```python
from build123d import *

# Parameters (mm, degrees)
F0_W     = 5.08
F0_H     = 5.08
F1_DEPTH = 2.54
F4_W     = 1.27
F4_H     = 3.048
F5_DEPTH = 5.08
F3_W     = 2.921
F3_H     = 1.27


with BuildPart() as f1:
    # F0 (on Right) → F1 (new body, symmetric)
    with BuildSketch(Plane.YZ):
        Rectangle(F0_W, F0_H)
    extrude(amount=F1_DEPTH, both=True)

    # F4 (on face) → F5 (cut, through all)
    with BuildSketch(Plane.YZ.offset(2.54)):
        Rectangle(F4_W, F4_H)
    extrude(amount=-F5_DEPTH, mode=Mode.SUBTRACT)

    # F6: sweep along a path in F2
    with BuildLine(Plane.XZ) as f6_path:
        Line((0, -2.54), (0, -6.096))
        Line((0, -6.096), (-10.541, -6.096))
        Line((-10.541, -6.096), (-10.541, 0))
        Line((-10.541, 0), (7.8415209427, 0))
    # F3 (on face) → F6 (sweep)
    with BuildSketch(Plane(origin=(0, 0, -2.54), x_dir=(1, 0, 0), z_dir=(0, 0, -1))):
        Rectangle(F3_W, F3_H)
    sweep(path=f6_path.line, transition=Transition.RIGHT)


solid = f1.part
```
Check sheet for the modelled part. Datum: model origin and axes. Units: mm. A direction names the side the tool comes from. Round coordinates to 2 decimals unless told otherwise and drop trailing zeros. Order: outer loops, then holes, each group sorted by start corner. A loop starts at its lowest first (then second) coordinate and runs counter-clockwise, first axis right, second up. Notation, with made-up numbers: (-14, 6.5) -> (1, 6.5) arc R3 cw to (1, 10.5) -> close; hole circle Ø11 at (70.25, -9). An arc over 180 degrees is marked (long way). One line per item, written item: value. Start each with the question number.
Q1. Cross-section at A-A (x = -4). Record the boundary of the cut face in (y, z) (1 decimal).
Q2. Thickness scan on line 1 (X direction, y = -0.25, z = -2); line 2 (Y direction, x = -9, z = -0.25) (3 decimals); line 3 (Z direction, x = -4.5, y = 0.35). Record the ranges inside material, lowest first.
Q3. Mould release check, pull along Z, two halves, no side actions. Record for faces 6 (the face through (-5, 0, -7.556)), 7 (the face through (-5, 0, -4.636)), 8 (the face through (-1.46, 0, -4)), 9 (the face through (-7, -0.635, -5)): pulls with the +Z half, pulls with the -Z half, needs draft (parallel to the pull), parting line crosses it, or undercut.
Q4. Cross-section at B-B (y = -0.2). Record the boundary of the cut face in (x, z).
Q5. Cross-section at D-D (x = -0.25). Give the number of separate pieces and of enclosed holes in the cut face, and give its area (3 significant figures).
Q6. Cross-section at C-C (z = -1). Record the boundary of the cut face in (x, y) (1 decimal).
Q7. Gauge pin test, flat ends, axial feed: pin 1 Ø4.5 at (x, z) = (-8, -2.5) entering from -Y (3 decimals); pin 2 Ø1 at (y, z) = (0.5, -4.5) entering from +X; pin 3 Ø1 at (x, y) = (4, -1) entering from +Z. Record the tip position at first contact, or that the pin passes through.
Q8. Set-up check for faces 1 (the face through (1.46, 0, -5)), 2 (the face through (-7, 0.635, -5)), 3 (the face through (-9.08, 0, -3)), 4 (the face through (5, -0.635, 0)), 5 (the face through (5, 0.635, 0)): record each of +Z, -Z, +X, -X, +Y, -Y from which the full face is reachable in a straight line by a thin tool's end or side.
Completed:
1. outline: (-0.6, -7.6) -> (0.6, -7.6) -> (0.6, -4.6) -> (-0.6, -4.6) -> close; (-0.6, -1.5) -> (0.6, -1.5) -> (0.6, 1.5) -> (-0.6, 1.5) -> close
2. line 1: x = -12 to -9.08, -2.54 to 2.54
2. line 2: y = -0.635 to 0.635
2. line 3: z = -7.56 to -4.64, -1.46 to 1.46
3. face 6: pulls with the -Z half
3. face 7: undercut
3. face 8: undercut
3. face 9: needs draft
4. outline: (-12, -7.56) -> (1.46, -7.56) -> (1.46, -2.54) -> (2.54, -2.54) -> (2.54, -1.52) -> (-2.54, -1.52) -> (-2.54, -2.54) -> (-1.46, -2.54) -> (-1.46, -4.64) -> (-9.08, -4.64) -> (-9.08, -1.46) -> (7.84, -1.46) -> (7.84, 1.46) -> (-12, 1.46) -> close; (-2.54, 1.52) -> (2.54, 1.52) -> (2.54, 2.54) -> (-2.54, 2.54) -> close
5. separate pieces: 1
5. enclosed holes: 2
5. area: 32.0 mm²
6. outline: (-12, -0.6) -> (-2.5, -0.6) -> (-2.5, -2.5) -> (2.5, -2.5) -> (2.5, -0.6) -> (7.8, -0.6) -> (7.8, 0.6) -> (2.5, 0.6) -> (2.5, 2.5) -> (-2.5, 2.5) -> (-2.5, 0.6) -> (-12, 0.6) -> close
7. pin 1: stops at y = -0.635
7. pin 2: stops at x = 1.46
7. pin 3: stops at z = 1.46
8. face 1: -Z, +X, +Y, -Y
8. face 2: -Z, -X, +Y
8. face 3: +Y, -Y
8. face 4: +Z, -Z, +X, -Y
8. face 5: +Z, -Z, +X, +Y
